Could you check a few things on this model? Use its own coordinates, in mm. A direction names the side the tool comes from. Round coordinates to 2 decimals unless told otherwise and drop trailing zeros. Write each loop counter-clockwise with the first axis right and the second up, starting at its lowest first coordinate (ties: lowest second). Pieces come first, ordered by that corner, then holes. Notation, with made-up numbers: M 30,18 L 66,18 A15 ccw 66,43 Z; hole C 64,-22.75 d1. An arc over 180 degrees is marked long. One line per item, written item: value. Start each with the question number.
(1) I want a section at A-A on x = 0. Please give me the cut outline in (y, z), and give its area (3 significant figures).
(2) Which directions (+Z, -Z, +X, -X, +Y, -Y) give clear straight access to the entire face, cutting with the end or side of a thin tool? Please do faces 1 (the face through (0, -164, 2)), 2 (the face through (0, -56, -2)), 3 (the face through (0, -188.87, 0)).
(3) I want a section at C-C on y = -162.5. Please give me the cut outline in (x, z).
(4) I want a section at B-B on z = 0. Please give me the cut outline in (x, y).
(5) I want a section at D-D on y = -130. Please give me the cut outline in (x, z).
(6) Thinking about a two-plate mould opening in Z: for faces 4 (the face through (-2.2, -52.07, 1)), 5 (the face through (0, -58.07, 0)), 6 (the face through (0.763, -122.747, 3.437)), which applies, released by +Z, released by -Z, zero draft, split by the parting line, or undercut?
(7) I'm going to push flat-ended pins straight in: pin 1 Ø3 at (x, y) = (1, -153.5) entering from +Z; pin 2 Ø2 at (x, y) = (-3.5, -147.5) entering from +Z; pin 3 Ø3 at (y, z) = (-135, -1) entering from -X; pin 4 Ø1 at (x, y) = (1, -112) entering from +Z. Where does each tip first touch, or does it pass through?
(8) If I drill on L1, parallel to Z at x = 0, y = -54.25; L2, parallel to Y at x = -1.75, z = -0.75; L3, parallel to X at y = -60, z = 3, over which ranges is the centre line in solid material (lowest first)?
```python
from build123d import *

# Parameters (mm, degrees)
SKETCH3_R          = 2.8067
CUT_EXTRUDE1_DEPTH = 12
CHAMFER1_SIZE      = 0.4
CHAMFER1_SIZE2     = 1.098990968
SKETCH4_R          = 2
CUT_EXTRUDE2_DEPTH = 6
CHAMFER2_SIZE      = 1
CHAMFER2_SIZE2     = 0.140540835


with BuildPart() as part:
    # Sketch1 → Revolve1 (revolve)
    with BuildSketch(Plane.XY, mode=Mode.PRIVATE) as revolve1_sk:
        Polygon((0, 95.25), (15.875, 95.25), (15.875, 0), (6.352863958, 0), (6.352863958, -38.836595706), (7.9248, -44.181178248), (7.9248, -52.07), (0, -52.07), align=None)
    revolve(revolve1_sk.sketch.rotate(Axis((0, 95.25, 0), (0, -1, 0)), 180), axis=Axis((0, 95.25, 0), (0, -1, 0)))

    # Sketch3 → Cut-Extrude1 (cut)
    with BuildSketch(Plane.XZ.offset(52.07)):
        Circle(SKETCH3_R)
    extrude(amount=-CUT_EXTRUDE1_DEPTH, mode=Mode.SUBTRACT)

    # Chamfer1
    chamfer1_edges = [part.edges().sort_by_distance(p)[0] for p in [
        (-2.8067, -52.07, 0),
    ]]
    chamfer1_side = [part.faces().sort_by_distance(p)[0] for p in [
        (7.700652807, -52.07, 0),
    ]]
    chamfer(chamfer1_edges, length=CHAMFER1_SIZE, length2=CHAMFER1_SIZE2, reference=chamfer1_side[0])


with BuildPart() as body_2:
    # Sketch2 → Revolve2 (revolve)
    with BuildSketch(Plane.XY, mode=Mode.PRIVATE) as revolve2_sk:
        Polygon((0, -52.07), (0, -188.87), (2, -188.87), (2, -138.87), (5, -107.07), (5, -52.07), align=None)
    revolve(revolve2_sk.sketch.rotate(Axis((0, -52.07, 0), (0, -1, 0)), 180), axis=Axis((0, -52.07, 0), (0, -1, 0)))

    # Sketch4 → Cut-Extrude2 (cut)
    with BuildSketch(Plane(origin=(0, -52.07, 0), x_dir=(1, 0, 0), z_dir=(0, 1, 0))):
        with Locations(Location((0, 0, 0), (0, 0, 180))):
            Circle(SKETCH4_R)
    extrude(amount=-CUT_EXTRUDE2_DEPTH, mode=Mode.SUBTRACT)

    # Chamfer2
    chamfer2_edges = [body_2.edges().sort_by_distance(p)[0] for p in [
        (2, -52.07, 0),
    ]]
    chamfer2_side = [body_2.faces().sort_by_distance(p)[0] for p in [
        (2, -55.07, 0),
    ]]
    chamfer(chamfer2_edges, length=CHAMFER2_SIZE, length2=CHAMFER2_SIZE2, reference=chamfer2_side[0])


solid = body_2.part
```
Found:
1. outline: M -188.87,-2 L -138.87,-2 L -107.07,-5 L -52.07,-5 L -52.07,-2.14 L -53.07,-2 L -58.07,-2 L -58.07,2 L -53.07,2 L -52.07,2.14 L -52.07,5 L -107.07,5 L -138.87,2 L -188.87,2 Z
1. area: 948 mm²
2. face 1: -Y
2. face 2: +Y
2. face 3: +Z, -Z, +X, -X, -Y
3. outline: C 0,0 d4
4. outline: M -5,-107.07 L -2,-138.87 L -2,-188.87 L 2,-188.87 L 2,-138.87 L 5,-107.07 L 5,-52.07 L 2.14,-52.07 L 2,-53.07 L 2,-58.07 L -2,-58.07 L -2,-53.07 L -2.14,-52.07 L -5,-52.07 Z
5. outline: C 0,0 d5.67
6. face 4: zero draft
6. face 5: undercut
6. face 6: split by the parting line
7. pin 1: stops at z = 2
7. pin 2: passes through
7. pin 3: stops at x = -2.48
7. pin 4: stops at z = 4.52
8. L1: z = -5 to -2, 2 to 5
8. L2: y = -188.87 to -58.07
8. L3: x = -4 to 4
